```python
from build123d import *

# Parameters (mm, degrees)
EXTRUDE_2_DEPTH     = 42
SKETCH_4_R          = 2.1
CUT_EXTRUDE_2_DEPTH = 42
SKETCH_5_R          = 2.1
CUT_EXTRUDE_3_DEPTH = 42


with BuildPart() as part:
    # 草图1 → 凸台-拉伸2 (new body)
    with BuildSketch(Plane.XY):
        Polygon((19, 0), (0, 0), (0, 19), align=None)
    extrude(amount=EXTRUDE_2_DEPTH)

    # 草图4 → 切除-拉伸2 (cut)
    with BuildSketch(Plane(origin=(0, 0, 0), x_dir=(-1, 0, 0), z_dir=(0, -1, 0))):
        with Locations(Location((-10.5, -32.75, 0), (0, 0, 90))):
            Circle(SKETCH_4_R)
        with Locations(Location((-10.5, -9.25, 0), (0, 0, 180))):
            Circle(SKETCH_4_R)
    extrude(amount=-CUT_EXTRUDE_2_DEPTH, mode=Mode.SUBTRACT)

    # 草图5 → 切除-拉伸3 (cut)
    with BuildSketch(Plane.ZY):
        with Locations((32.75, 10.5)):
            Circle(SKETCH_5_R)
        with Locations(Location((9.25, 10.5, 0), (0, 0, 331.563109851))):
            Circle(SKETCH_5_R)
    extrude(amount=-CUT_EXTRUDE_3_DEPTH, mode=Mode.SUBTRACT)


solid = part.part
```
Geometry check sheet. Reference: the model listing, model coordinates, mm. Coordinates: 2 decimals unless noted, no trailing zeros. Order: outer loops, then holes, each group sorted by start corner. A loop starts at its lowest first (then second) coordinate and runs counter-clockwise, first axis right, second up. Notation, with made-up numbers: M 38,19.5 L 93,19.5 A12 cw 93,25.5 Z; hole C 86,-34.75 d9. An arc over 180 degrees is marked long. Answer as a JSON object with one key per item and string values.
Q1. Depth check by flat-ended pin: pin 1 Ø1.5 at (y, z) = (12.5, 35) entering from +X; pin 2 Ø6.5 at (x, z) = (10.5, 9.25) entering from +Y; pin 3 Ø3 at (x, z) = (13, 33.5) entering from +Y; pin 4 Ø1.5 at (x, z) = (15, 14.5) entering from -Y. Enter the tip coordinate at first touch or a pass-through.
Results are:
{"pin 1": "stops at x = 7.25", "pin 2": "stops at y = 11.04", "pin 3": "stops at y = 7.2", "pin 4": "stops at y = 0"}
Q2. Cross-section at B-B on x = 10.5. Record the cut outline in (y, z).
Results are:
{"outline": "M 0,0 L 8.5,0 L 8.5,7.15 L 0,7.15 Z; M 0,11.35 L 8.5,11.35 L 8.5,30.65 L 0,30.65 Z; M 0,34.85 L 8.5,34.85 L 8.5,42 L 0,42 Z"}
Q3. Release check for a two-part mould opening along X. For faces 1 (the cylindrical face through (8.4, 3.6, 9.3)), 2 (the flat face through (5, 5, 42)), 3 (the flat face through (9, 10, 21)) record: released by +X, released by -X, zero draft, split by the parting line, or undercut.
Results are:
{"face 1": "undercut", "face 2": "zero draft", "face 3": "released by +X"}
Q4. Cross-section at A-A on z = 9.25. Record the cut outline in (x, y), and give its area (3 significant figures).
Results are:
{"outline": "M 0,0 L 8.4,0 L 8.4,8.4 L 0,8.4 Z; M 0,12.6 L 6.4,12.6 L 0,19 Z; M 12.6,0 L 19,0 L 12.6,6.4 Z", "area": "112 mm²"}
Q5. Cross-section at D-D on y = 5. Record the cut outline in (x, z).
Results are:
{"outline": "M 0,0 L 14,0 L 14,42 L 0,42 Z; hole C 10.5,9.25 d4.2; hole C 10.5,32.75 d4.2"}
Q6. Scan lines: line 1 (Z direction, x = 3.5, y = 10.75); line 2 (Z direction, x = 4.5, y = 12); line 3 (Y direction, x = 3.25, z = 32.75). Record each from-to range of solid material in increasing order.
Results are:
{"line 1": "z = 0 to 7.16, 11.34 to 30.66, 34.84 to 42", "line 2": "z = 0 to 7.78, 10.72 to 31.28, 34.22 to 42", "line 3": "y = 0 to 8.4, 12.6 to 15.75"}
